Can you work these out from the model? Positions are in its coordinate system, mm. A direction names the side the tool comes from. Coordinates: 2 decimals unless noted, no trailing zeros. Return JSON: item names as keys, results as strings. Group by question number.
```python
from build123d import *

# Parameters (mm, degrees)
SKETCH1_W                     = 7
SKETCH1_H                     = 35
BOSS_EXTRUDE1_DEPTH           = 1.7
BOSS_EXTRUDE1_TAPER           = 5
BOSS_EXTRUDE1_OTHER_WAY_DEPTH = 1.7
BOSS_EXTRUDE1_OTHER_WAY_TAPER = 5
SKETCH2_W                     = 1.5
SKETCH2_H                     = 0.41
CUT_EXTRUDE1_DEPTH            = 1.7


with BuildPart() as part:
    # Sketch1 → Boss-Extrude1 (new body)
    with BuildSketch(Plane(origin=(0, 0, 0), x_dir=(1, 0, 0), z_dir=(0, 1, 0))):
        with Locations((3.5, 17.5)):
            Rectangle(SKETCH1_W, SKETCH1_H)
    extrude(amount=BOSS_EXTRUDE1_DEPTH, taper=BOSS_EXTRUDE1_TAPER)

    # Sketch1 → Boss-Extrude1 other way (add)
    with BuildSketch(Plane(origin=(0, 0, 0), x_dir=(1, 0, 0), z_dir=(0, 1, 0))):
        with Locations((3.5, 17.5)):
            Rectangle(SKETCH1_W, SKETCH1_H)
    extrude(amount=-BOSS_EXTRUDE1_OTHER_WAY_DEPTH, taper=BOSS_EXTRUDE1_OTHER_WAY_TAPER)

    # Sketch2 → Cut-Extrude1 (cut)
    with BuildSketch(Plane(origin=(6.946827136, -0.607768622, 0), x_dir=(0, 0, -1), z_dir=(0.996194698, -0.087155743, 0))):
        with Locations((1.25, 0.405090199)):
            Rectangle(SKETCH2_W, SKETCH2_H)
        with Locations((3.75, 0.405090199)):
            Rectangle(SKETCH2_W, SKETCH2_H)
        with Locations((6.25, 0.405090199)):
            Rectangle(SKETCH2_W, SKETCH2_H)
        with Locations((8.75, 0.405090199)):
            Rectangle(SKETCH2_W, SKETCH2_H)
        with Locations((11.25, 0.405090199)):
            Rectangle(SKETCH2_W, SKETCH2_H)
        with Locations((13.75, 0.405090199)):
            Rectangle(SKETCH2_W, SKETCH2_H)
        with Locations((16.25, 0.405090199)):
            Rectangle(SKETCH2_W, SKETCH2_H)
        with Locations((18.75, 0.405090199)):
            Rectangle(SKETCH2_W, SKETCH2_H)
        with Locations((21.25, 0.405090199)):
            Rectangle(SKETCH2_W, SKETCH2_H)
        with Locations((23.75, 0.405090199)):
            Rectangle(SKETCH2_W, SKETCH2_H)
        with Locations((26.25, 0.405090199)):
            Rectangle(SKETCH2_W, SKETCH2_H)
        with Locations((28.75, 0.405090199)):
            Rectangle(SKETCH2_W, SKETCH2_H)
        with Locations((31.25, 0.405090199)):
            Rectangle(SKETCH2_W, SKETCH2_H)
        with Locations((33.75, 0.405090199)):
            Rectangle(SKETCH2_W, SKETCH2_H)
    cut_extrude1 = extrude(amount=-CUT_EXTRUDE1_DEPTH, mode=Mode.SUBTRACT)

    # Mirror1: Cut-Extrude1 across plane
    add(cut_extrude1.mirror(Plane(origin=(3.5, 0, 0), x_dir=(0, 0, 1), z_dir=(1, 0, 0))), mode=Mode.SUBTRACT)


solid = part.part
```
1) Suppose I cut it at A-A, the plane x = 1. Give the number of separate pieces and of enclosed holes in the cut face, then the cut area to 3 significant figures.
2) For pin 1 (1 mm diameter, centred on y = -1, z = -31.5, fed in from -X), with a flat end and sliding along its axis, tell me the tip position at first contact or that it passes through.
3) For faces 1 (the face through (6.129, -0.335, -21.24)), 2 (the face through (3, 1.7, -17)), 3 (the face through (6.165, 0.073, -3.74)), 4 (the face through (0.871, -0.335, -33.74)), which set-ups out of +Z, -Z, +X, -X, +Y, -Y let a thin tool reach every point of the face, with its end or its side?
4) If we mould it in two halves opening along Z, with no side actions, what happens to faces 5 (the face through (3, -1.7, -17)), 6 (the face through (0.871, -0.335, -1.24))? For each: +Z half, -Z half, draft (parallel to the pull), parting line (faces both ways), or undercut.
5) If I drill on line 1 (Z direction, x = 3, y = 0.1); line 2 (Z direction, x = 3.5, y = -0.7); line 3 (X direction, y = -0.8, z = -3.5), over which ranges is the centre line in solid material (lowest first)? Write a range as from..to.
Returned:
{
 "1": {"separate pieces": "1", "enclosed holes": "14", "area": "110 mm²"},
 "2": {"pin 1": "stops at x = 0.04"},
 "3": {"face 1": "+X", "face 2": "+Z, -Z, +X, -X, +Y", "face 3": "none", "face 4": "-X"},
 "4": {"face 5": "draft", "face 6": "undercut"},
 "5": {"line 1": "z = -34.99..-0.01", "line 2": "z = -34.94..-0.06", "line 3": "x = 0.07..6.93"}
}
